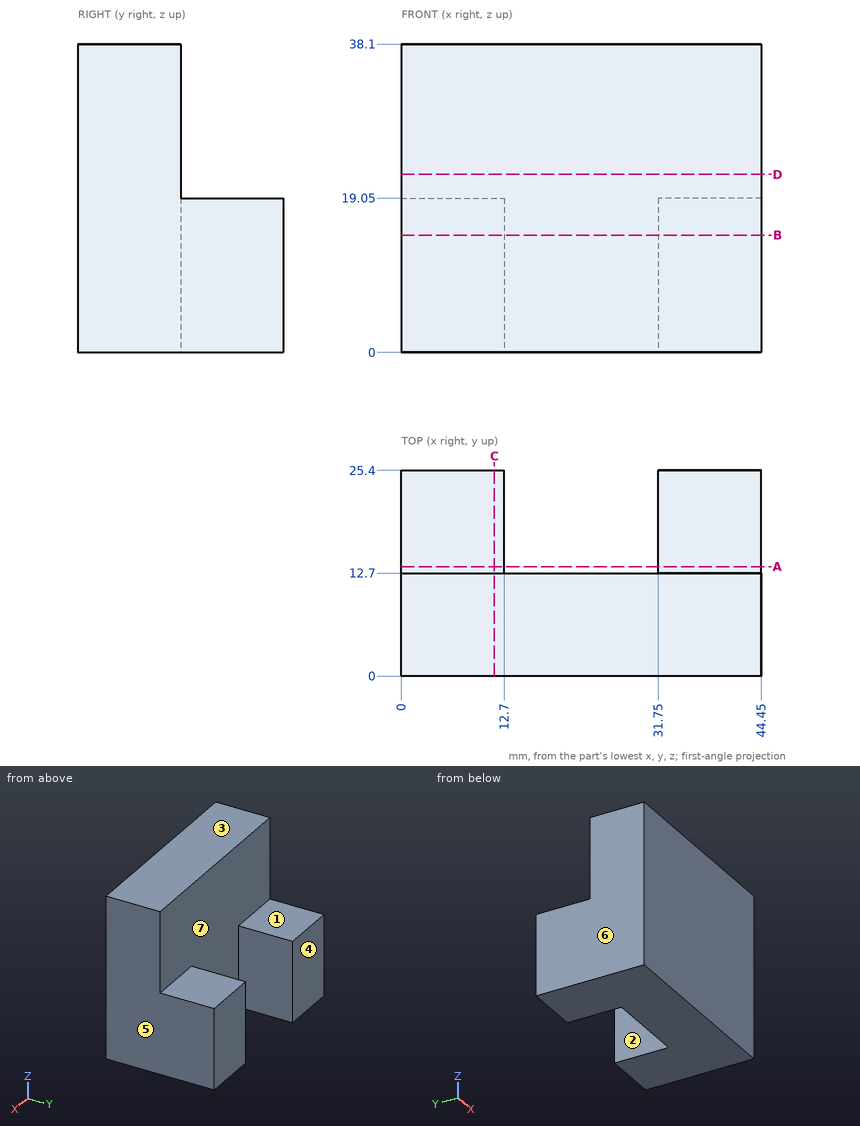
Design review of the part shown in the three views and the two pictorial views. Dimensions are in mm from the part's minimum x, y and z. A direction names the side the tool comes from. Round coordinates to 2 decimals unless told otherwise and drop trailing zeros. Order: outer loops, then holes, each group sorted by start corner. A loop starts at its lowest first (then second) coordinate and runs counter-clockwise, first axis right, second up.
Q1. Machinability: for the marked faces 1, 2 and 3, which of the approach directions +Z, -Z, +X, -X, +Y, -Y give a long, thin tool a straight path to every point of the face, cutting with its end or side? Answer none if there is none.
Findings below:
face 1: +Z, +X, -X, +Y
face 2: +Z, -Z, +Y
face 3: +Z, +X, -X, +Y, -Y
Q2. We need section C-C, the plane x = 11.5. Give the boundary of the cut face in (y, z).
Findings below:
outline: (0, 0) - (25.4, 0) - (25.4, 19.05) - (12.7, 19.05) - (12.7, 38.1) - (0, 38.1) - close
Q3. We need section B-B, the plane z = 14.5. Give the boundary of the cut face in (x, y).
Findings below:
outline: (0, 0) - (44.45, 0) - (44.45, 25.4) - (31.75, 25.4) - (31.75, 12.7) - (12.7, 12.7) - (12.7, 25.4) - (0, 25.4) - close
Q4. We need section D-D, the plane z = 22. Give the boundary of the cut face in (x, y).
Findings below:
outline: (0, 0) - (44.45, 0) - (44.45, 12.7) - (0, 12.7) - close
Q5. Insertion check: P1, Ø4, axis at x = 35.5, y = 18, coming from the +Z side. The pin has a flat end and moves straight along its axis. Give the tip position at first contact, or say it passes through.
Findings below:
P1: stops at z = 19.05
Q6. Wall thickness on line 1 (Y direction, x = 38, z = 34.5); line 2 (X direction, y = 18.25, z = 3); line 3 (Z direction, x = 33, y = 16.25): over which ranges is each line inside the solid? List them lowest first.
Findings below:
line 1: y = 0 to 12.7
line 2: x = 0 to 12.7, 31.75 to 44.45
line 3: z = 0 to 19.05
Q7. We need section A-A, the plane y = 13.5. Give the boundary of the cut face in (x, z).
Findings below:
outline: (0, 0) - (12.7, 0) - (12.7, 19.05) - (0, 19.05) - close; (31.75, 0) - (44.45, 0) - (44.45, 19.05) - (31.75, 19.05) - close
Q8. Mouldability with a two-part tool opening along X and no side actions: class the marked faces 4, 5, 6 and 7 as pulls with the +X half, pulls with the -X half, needs draft (parallel to the pull), parting line crosses it, or undercut.
Findings below:
face 4: needs draft
face 5: pulls with the +X half
face 6: pulls with the -X half
face 7: undercut
